Build history of the part. All positions in model axes, mm. Face numbers are marked on the shaded views. Round coordinates to 2 decimals unless told otherwise and drop trailing zeros. Write each loop counter-clockwise with the first axis right and the second up, starting at its lowest first coordinate (ties: lowest second). Pieces come first, ordered by that corner, then holes. Notation, with made-up numbers: (26.5, -2) -> (83.5, -2) arc R27 cw to (83.5, 16) -> close; hole circle Ø11 at (61, 1). An arc over 180 degrees is marked (long way). Answer in a Markdown table with one row per item. Add a question column.
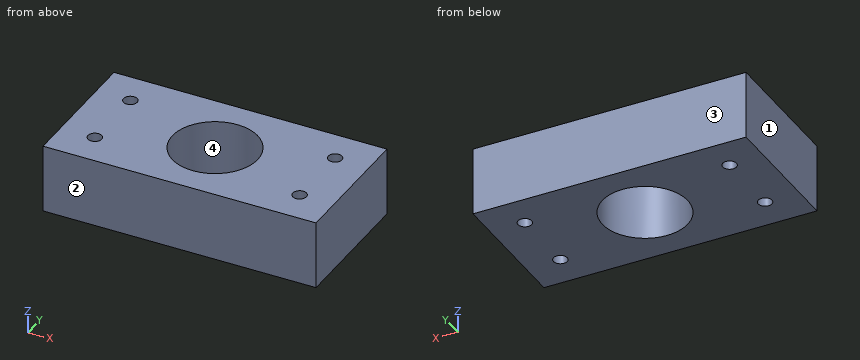
from build123d import *

# Parameters (mm, degrees)
SKETCH1_W               = 101.6
SKETCH1_H               = 25.4
BOSS_EXTRUDE1_DEPTH     = 25.4
CUT_EXTRUDE1_REACH      = 64.217
SKETCH2_R               = 15.875
F_1_4_20_TAPPED_HOLE1_D = 5.1054


with BuildPart() as part:
    # Sketch1 → Boss-Extrude1 (new, symmetric)
    with BuildSketch(Plane(origin=(0, 0, 0), x_dir=(1, 0, 0), z_dir=(0, 1, 0))):
        Rectangle(SKETCH1_W, SKETCH1_H)
    extrude(amount=BOSS_EXTRUDE1_DEPTH, both=True)

    # Sketch2 → Cut-Extrude1 (cut, up to next)
    with BuildSketch(Plane.XY.offset(12.7), mode=Mode.PRIVATE) as cut_extrude1_sk1:
        Circle(SKETCH2_R)
    cut_extrude1_tool1 = extrude(cut_extrude1_sk1.sketch, amount=-CUT_EXTRUDE1_REACH, mode=Mode.PRIVATE) & part.part
    add(cut_extrude1_tool1.solids().sort_by_distance((0, 0, 12.7))[0], mode=Mode.SUBTRACT)

    # 1/4-20 Tapped Hole1 (through all)
    with Locations(Plane.XY.offset(12.7)):
        with Locations((-38.1, 12.7), (-38.1, -12.7), (38.1, 12.7), (38.1, -12.7)):
            Hole(F_1_4_20_TAPPED_HOLE1_D / 2)


solid = part.part
(1) Saw through at A-A (x = 38.1). List the corners of the cut face in (y, z).
(2) Saw through at B-B (z = -0.25). List the corners of the cut face in (x, y) (3 decimals), plus the area to 3 significant figures.
(3) Mould opens along Y. For the marked faces 1, 2, 3 and 4 say: pulls with the +Y half, pulls with the -Y half, needs draft (parallel to the pull), parting line crosses it, or undercut.
(4) Saw through at D-D (x = 0). List the corners of the cut face in (y, z) (3 decimals).
(5) Drop flat-ended pins along their axis: P1, Ø4, axis at x = 38.1, y = 12.7, coming from the +Z side; P2, Ø5, axis at x = -14, y = -1, coming from the +Z side. Give the stop position or say it passes through.
(6) Probe line 1 along Y through (x, z) = (38.1, -3.75); line 2 along Y through (x, z) = (0, -1.25) (3 decimals); line 3 along X through (y, z) = (13, 7). List the from-to ranges inside material, lowest first.
(7) Saw through at C-C (y = 0). List the corners of the cut face in (x, z) (3 decimals), plus the area to 3 significant figures.
Answer sheet:
| question | item | result |
|---|---|---|
| 1 | outline | (-25.4, -12.7) -> (-15.25, -12.7) -> (-15.25, 12.7) -> (-25.4, 12.7) -> close; (-10.15, -12.7) -> (10.15, -12.7) -> (10.15, 12.7) -> (-10.15, 12.7) -> close; (15.25, -12.7) -> (25.4, -12.7) -> (25.4, 12.7) -> (15.25, 12.7) -> close |
| 2 | outline | (-50.8, -25.4) -> (50.8, -25.4) -> (50.8, 25.4) -> (-50.8, 25.4) -> close; hole circle Ø5.105 at (-38.1, -12.7); hole circle Ø5.105 at (-38.1, 12.7); hole circle Ø31.75 at (0, 0); hole circle Ø5.105 at (38.1, -12.7); hole circle Ø5.105 at (38.1, 12.7) |
| 2 | area | 4,290 mm² |
| 3 | face 1 | needs draft |
| 3 | face 2 | pulls with the -Y half |
| 3 | face 3 | pulls with the +Y half |
| 3 | face 4 | undercut |
| 4 | outline | (-25.4, -12.7) -> (-15.875, -12.7) -> (-15.875, 12.7) -> (-25.4, 12.7) -> close; (15.875, -12.7) -> (25.4, -12.7) -> (25.4, 12.7) -> (15.875, 12.7) -> close |
| 5 | P1 | passes through |
| 5 | P2 | stops at z = 12.7 |
| 6 | line 1 | y = -25.4 to -15.25, -10.15 to 10.15, 15.25 to 25.4 |
| 6 | line 2 | y = -25.4 to -15.875, 15.875 to 25.4 |
| 6 | line 3 | x = -50.8 to -40.64, -35.56 to -9.11, 9.11 to 35.56, 40.64 to 50.8 |
| 7 | outline | (-50.8, -12.7) -> (-15.875, -12.7) -> (-15.875, 12.7) -> (-50.8, 12.7) -> close; (15.875, -12.7) -> (50.8, -12.7) -> (50.8, 12.7) -> (15.875, 12.7) -> close |
| 7 | area | 1,770 mm² |
